Work out the finished part from the listing and answer in its coordinate system (mm). A direction names the side the tool comes from. Round coordinates to 2 decimals unless told otherwise and drop trailing zeros. Write each loop counter-clockwise with the first axis right and the second up, starting at its lowest first coordinate (ties: lowest second). Pieces come first, ordered by that corner, then holes. Notation, with made-up numbers: (-23, -1.75) -> (27, -1.75) arc R20 ccw to (27, 17.25) -> close; hole circle Ø1 at (83.5, 71.25). An arc over 180 degrees is marked (long way). One line per item, written item: value.
Autodesk Inventor part; units mm, degrees
ref_plane "YZ Plane" through (0, 0, 0) normal (1, 0, 0) x (0, 1, 0)
ref_plane "XZ Plane" through (0, 0, 0) normal (0, 1, 0) x (-1, 0, 0)
ref_plane "XY Plane" through (0, 0, 0) normal (0, 0, 1) x (1, 0, 0)
sketch "Sketch1" plane through (0, 0, 0) normal (1, 0, 0) x (0, 1, 0)
  line L0 (0, 116.2) -> (0, -116.2)
  line L1 (-61.6, 0) -> (61.6, 0)
  line L2 (44, 83) -> (-44, 83)
  line L3 (-44, 83) -> (-44, -83)
  line L4 (-44, -83) -> (44, -83)
  line L5 (44, -83) -> (44, 83)
  point P0 (0, 0)
  dimension "d0" = 166
  dimension "d1" = 88
extrude "Extrusion1" add sketch "Sketch1" along normal blind 32
sketch "Sketch2" plane through (32, 0, 0) normal (1, 0, 0) x (0, 0, -1)
  line L0 (-116.2, 0) -> (116.2, 0)
  line L1 (0, -61.6) -> (0, 61.6)
  circle A0 centre (0, 0) radius 44
  arc A1 (24.7538, 3.5) -> (24.7538, -3.5) centre (0, 0) ccw
  line L2 (25, 0) -> (29, 0)
  line L3 (29, 0) -> (29, 3.5)
  line L4 (29, 3.5) -> (24.7538, 3.5)
  arc A2 (24.7538, 3.5) -> (24.7538, -3.5) centre (0, 0) ccw
  line L5 (29, 0) -> (29, -3.5)
  line L6 (29, -3.5) -> (24.7538, -3.5)
  dimension "d4" = 88
  dimension "d5" = 50
  dimension "d6" = 4
  dimension "d7" = 3.5
extrude "Extrusion2" add sketch "Sketch2" along normal blind 58 contours L3 L4 A1 L1 A0 L0 | L0 A0 L1 A1 L6 L5 | A1 L1 A0 L0 | L0 A0 L1 A1
sketch "Sketch3" plane through (0, 0, 0) normal (-1, 0, 0) x (0, 0, 1)
  line L0 (-116.2, 0) -> (116.2, 0)
  line L1 (0, 61.6) -> (0, -61.6)
  line L2 (-83, 44) -> (83, 44)
  line L3 (83, -44) -> (-83, -44)
  line L4 (-83, 44) -> (-55, 44)
  line L5 (-55, 44) -> (-55, -44)
  line L6 (-55, -44) -> (-83, -44)
  line L7 (-83, -44) -> (-83, 44)
  line L8 (0, 44) -> (83, 44)
  line L9 (83, 44) -> (55, 44)
  line L10 (55, 44) -> (55, -44)
  line L11 (55, -44) -> (83, -44)
  line L12 (83, -44) -> (83, 44)
  point P0 (0, 0)
  dimension "d10" = 28
  dimension "d11" = 28
extrude "Extrusion3" add sketch "Sketch3" along normal blind 98 contours L7 L2 L5 L0 | L0 L5 L3 L7 | L10 L2 L12 L0 | L0 L12 L3 L10
sketch "Sketch4" plane through (32, -44, 83) normal (0, 0, 1) x (1, 0, 0)
  point P0 (-32, 44)
sketch "Sketch5" plane through (32, -44, 83) normal (0, 0, 1) x (1, 0, 0)
  circle A0 centre (-92, 44) radius 38
  line L0 (-92, 6) -> (-32, 0)
  line L1 (-130, 0) -> (0, 0)
  line L2 (-32, 88) -> (-32, 0)
  line L3 (-32, 88) -> (-92, 82)
  line L4 (0, 88) -> (-130, 88)
  line L5 (-32, 88) -> (-130, 88)
  line L6 (-130, 0) -> (-130, 88)
  line L7 (-130, 88) -> (-130, 0)
  line L8 (-130, 0) -> (-32, 0)
  point P0 (-32, 44)
  dimension "d14" = 76
extrude "Extrusion4" cut sketch "Sketch5" against normal through all contours A0 L6 L4 L3 | L0 L1 L6 A0
sketch "Sketch6" plane through (32, -44, 83) normal (0, 0, 1) x (1, 0, 0)
  arc A0 (-92, 82) -> (-92, 6) centre (-92, 44) ccw
  circle A1 centre (-92, 44) radius 16
  point P0 (-32, 44)
  dimension "d17" = 32
extrude "Extrusion5" cut sketch "Sketch6" against normal through all
properties part number "Fork 2 Off" material "Stainless Steel"
(1) A tool of negligible diameter and unlimited length cuts with its end or side. For faces 4 (the face through (-37, 1, 55)), 5 (the face through (-30, 41, 69)), 6 (the face through (61, 0, -29)), from which of +Z, -Z, +X, -X, +Y, -Y can it reach the whole face along a straight path? Write none if from no direction.
Reported:
face 4: -X, +Y, -Y
face 5: +Z, -Z, -X, +Y
face 6: +X
(2) Flat-ended cylindrical pins translate along their axes: pin 1 Ø1.3 at (x, z) = (57, -27) entering from -Y; pin 2 Ø25 at (y, z) = (21.5, 54) entering from +X; pin 3 Ø3.5 at (x, y) = (58.5, 0) entering from +Z; pin 4 Ø1 at (y, z) = (-28, 34) entering from +X. Find the tip coordinate at first contact, or state that the pin passes through.
Reported:
pin 1: stops at y = -35.24
pin 2: stops at x = 32
pin 3: stops at z = 44
pin 4: stops at x = 90
(3) Find section C-C on x = 70.5. Give the vertices of the cut face in (y, z), plus the area to 3 significant figures.
Reported:
outline: circle Ø88 at (0, 0); hole (-3.5, -29) -> (3.5, -29) -> (3.5, -24.75) arc R25 ccw (long way) to (-3.5, -24.75) -> close
area: 4,090 mm2
(4) Find section D-D on y = 35.5. Give the vertices of the cut face in (x, z).
Reported:
outline: (-73.56, -83) -> (32, -83) -> (32, -26) -> (90, -26) -> (90, 26) -> (32, 26) -> (32, 83) -> (-73.56, 83) -> (-73.56, 55) -> (0, 55) -> (0, -55) -> (-73.56, -55) -> close
(5) Consider probe 1 along Z at (x, y) = (-23, -14); probe 2 along Y at (x, z) = (-60, -61.5); probe 3 along Z at (x, y) = (57, 0). Determine where each line is inside the solid, lowest interval first.
Reported:
probe 1: z = -83 to -55, 55 to 83
probe 2: y = -38 to -16, 16 to 38
probe 3: z = -44 to -29, 25 to 44
(6) Find section A-A on x = -36. Give the vertices of the cut face in (y, z), plus the area to 3 significant figures.
Reported:
outline: (-40.4, -83) -> (40.4, -83) -> (40.4, -55) -> (-40.4, -55) -> close; (-40.4, 55) -> (40.4, 55) -> (40.4, 83) -> (-40.4, 83) -> close
area: 4,520 mm2
(7) Find section B-B on y = -12. Give the vertices of the cut face in (x, z), plus the area to 3 significant figures.
Reported:
outline: (-96.06, -83) -> (-70.58, -83) -> (-70.58, -55) -> (-96.06, -55) -> close; (-96.06, 55) -> (-70.58, 55) -> (-70.58, 83) -> (-96.06, 83) -> close; (-49.42, -83) -> (32, -83) -> (32, -42.33) -> (90, -42.33) -> (90, -21.93) -> (32, -21.93) -> (32, 21.93) -> (90, 21.93) -> (90, 42.33) -> (32, 42.33) -> (32, 83) -> (-49.42, 83) -> (-49.42, 55) -> (0, 55) -> (0, -55) -> (-49.42, -55) -> close
area: 11,900 mm2
(8) For a pull along Z with two mould halves and no side action, classify faces 1 (the face through (-19, -1, -83)), 2 (the face through (-37, 1, -55)), 3 (the face through (-75.985, 0.703, -68.804)) as pulls with the +Z half, pulls with the -Z half, needs draft (parallel to the pull), parting line crosses it, or undercut.
Reported:
face 1: pulls with the -Z half
face 2: undercut
face 3: needs draft
